Verification items for the finished model (mm, model axes). Face numbers are marked on the shaded views. A direction names the side the tool comes from. Give positions to 0.01 mm unless a question says otherwise; leave off trailing zeros. Order: outer loops, then holes, each group sorted by start corner. A loop starts at its lowest first (then second) coordinate and runs counter-clockwise, first axis right, second up. Notation, with made-up numbers: (-21.5, -20) - (-7.5, -20) arc R27 ccw to (-7.5, 8) - close; hole circle Ø10 at (34, -4.5). An arc over 180 degrees is marked (long way). Answer as a JSON object with one key per item and string values. Group by question number.
(1) Thickness scan on line 1 (Y direction, x = 0, z = 2.4); line 2 (Y direction, x = 0, z = 6); line 3 (Z direction, x = -3.75, y = 1.75). Record the ranges inside material, lowest first.
(2) Section check A-A (x = 0). Record the boundary of the cut face in (y, z), then the cut area to 3 significant figures.
(3) Depth check by flat-ended pin: pin 1 Ø5.5 at (x, y) = (0, 0) entering from +Z; pin 2 Ø2.5 at (x, y) = (-1, 7.5) entering from -Z; pin 3 Ø0.6 at (x, z) = (0.5, 0.5) entering from +Y; pin 4 Ø1 at (x, z) = (0.5, 1) entering from -Y. Enter the tip coordinate at first touch or a pass-through.
(4) Section check C-C (z = 3.75). Record the boundary of the cut face in (x, y).
(5) Section check B-B (z = 1.5). Record the boundary of the cut face in (x, y), then the cut area to 3 significant figures.
(6) Access from +Z, -Z, +X, -X, +Y, -Y to the whole of each face (thin tool, end or side, straight path). Record for the marked faces 1, 2 and 3.
(7) Section check D-D (y = -2.5). Record the boundary of the cut face in (x, z).
(8) Mould release check, pull along Z, two halves, no side actions. Record for the marked faces 4, 5 and 6: +Z half, -Z half, draft (parallel to the pull), parting line (faces both ways), or undercut.
Autodesk Inventor part; units mm, degrees
ref_plane "YZ Plane" through (0, 0, 0) normal (1, 0, 0) x (0, 1, 0)
ref_plane "XZ Plane" through (0, 0, 0) normal (0, 1, 0) x (-1, 0, 0)
ref_plane "XY Plane" through (0, 0, 0) normal (0, 0, 1) x (1, 0, 0)
sketch "Sketch1" plane through (0, 0, 0) normal (0, 0, 1) x (1, 0, 0)
  line L0 (7, 10) -> (-7, 10)
  line L1 (-7, 10) -> (-7, -10)
  line L2 (-7, -10) -> (7, -10)
  line L3 (7, -10) -> (7, 10)
  circle A0 centre (0, 0) radius 3.05
  point P0 (0, -10)
  point P1 (7, 0)
  dimension "d0" = 20
  dimension "d1" = 14
  dimension "d2" = 6.1
extrude "Extrusion1" add sketch "Sketch1" along normal blind 4.4
sketch "Sketch2" plane through (0, 0, 4.4) normal (0, 0, 1) x (1, 0, 0)
  circle A0 centre (0, 0) radius 3 construction
  circle A1 centre (0, 0) radius 7.5 construction
  circle A2 centre (0, 0) radius 3.05 construction
  line L0 (7, 10) -> (-7, 10)
  line L1 (-7, 10) -> (-7, -10)
  line L2 (-7, -10) -> (7, -10)
  line L3 (7, -10) -> (7, 10)
  circle A3 centre (0, 0) radius 7.6
  line L4 (7, -10) -> (7, 10)
  line L5 (7, 2.9597) -> (7, 10)
  line L6 (7, 10) -> (-7, 10)
  line L7 (7, 10) -> (-7, 10)
  line L8 (-7, 10) -> (-7, 2.9597)
  line L9 (-7, 10) -> (-7, -10)
  line L10 (-7, -2.9597) -> (-7, -10)
  line L11 (-7, -10) -> (7, -10)
  line L12 (7, -2.9597) -> (7, -10)
  dimension "d5" = 15.2
extrude "Extrusion2" add sketch "Sketch2" along normal blind 3 contours L3 A3 L1 L0 | L3 L2 L1 A3
sketch "Sketch4" plane through (0, 0, 0) normal (0, 0, -1) x (-1, 0, 0)
  circle A0 centre (0, 7.366) radius 1.15
  circle A1 centre (0, -7.366) radius 1.15
  circle A2 centre (0, 7.366) radius 1.5
  circle A3 centre (0, -7.366) radius 1.5
  point P0 (0, 0)
  dimension "d11" = 3
extrude "Extrusion4" cut sketch "Sketch4" against normal through all contours A0 | A1 | A2 | A3
sketch "Sketch3" plane through (0, 0, 0) normal (0, 0, -1) x (-1, 0, 0)
  circle A0 centre (0, 7.366) radius 1.15 construction
  circle A1 centre (0, -7.366) radius 1.15 construction
  line L0 (2.754, 7.366) -> (1.377, 4.981)
  line L1 (1.377, 4.981) -> (-1.377, 4.981)
  line L2 (-1.377, 4.981) -> (-2.754, 7.366)
  line L3 (-2.754, 7.366) -> (-1.377, 9.751)
  line L4 (-1.377, 9.751) -> (1.377, 9.751)
  line L5 (1.377, 9.751) -> (2.754, 7.366)
  line L6 (1.377, 9.751) -> (1.2332, 10)
  line L7 (-1.377, 9.751) -> (-1.2332, 10)
  line L8 (1.2332, 10) -> (-1.2332, 10)
  line L9 (-7, 10) -> (7, 10)
  point P0 (0, 0)
  dimension "d8" = 4.77
extrude "Extrusion3" cut sketch "Sketch3" against normal blind 2
sketch "Sketch5" plane through (-1.377, 4.981, 0) normal (0, 1, 0) x (1, 0, 0)
  line L0 (-1.377, 0) -> (-1.377, -2) construction
  line L1 (-1.377, 0) -> (-1.377, -1)
  arc A0 (-1.377, -1) -> (-1.377, 0) centre (-1.7436, -0.5) ccw
  point P0 (1.377, 0)
  point P1 (-1.377, -0.5)
  dimension "d15" = 0.62
  dimension "d16" = 0.3666
extrude "Extrusion5" add sketch "Sketch5" along normal blind 3
pattern_circular "Circular Pattern1" count 4 over 180 about axis through (0, 7.366, 0) along (0, 0, 1) of "Extrusion5"
mirror "Mirror1" about plane through (0, 0, 0) normal (0, 1, 0) of "Extrusion3", "Extrusion5", "Circular Pattern1"
chamfer "Chamfer1" distance 2 angle 45 4 edges at (-7, -10, 3.7) (-7, 10, 3.7) (7, 10, 3.7) (7, -10, 3.7)
properties part number "Arm1_BallCasterMount"
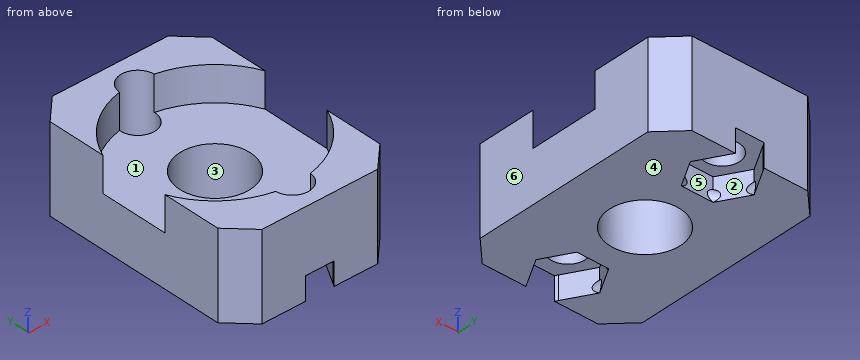
Solutions:
{
 "1": {"line 1": "y = -10 to -8.87, -5.87 to -3.05, 3.05 to 5.87, 8.87 to 10", "line 2": "y = -10 to -8.87, 8.87 to 10", "line 3": "z = 0 to 4.4"},
 "2": {"outline": "(-10, 2) - (-8.87, 2) - (-8.87, 7.4) - (-10, 7.4) - close; (-5.87, 2) - (-4.98, 2) - (-4.98, 0) - (-3.05, 0) - (-3.05, 4.4) - (-5.87, 4.4) - close; (3.05, 0) - (4.98, 0) - (4.98, 2) - (5.87, 2) - (5.87, 4.4) - (3.05, 4.4) - close; (8.87, 2) - (10, 2) - (10, 7.4) - (8.87, 7.4) - close", "area": "33.5 mm2"},
 "3": {"pin 1": "passes through", "pin 2": "stops at z = 2", "pin 3": "stops at y = 4.98", "pin 4": "stops at y = -4.98"},
 "4": {"outline": "(-7, -8) - (-5, -10) - (5, -10) - (7, -8) - (7, 8) - (5, 10) - (-5, 10) - (-7, 8) - close; hole circle Ø6.1 at (0, 0); hole circle Ø3 at (0, -7.37); hole circle Ø3 at (0, 7.37)"},
 "5": {"outline": "(-7, -8) - (-5, -10) - (-1.23, -10) - (-1.38, -9.75) - (-2.75, -7.37) - (-1.38, -4.98) - (1.38, -4.98) - (2.75, -7.37) - (1.38, -9.75) - (1.23, -10) - (5, -10) - (7, -8) - (7, 8) - (5, 10) - (1.23, 10) - (1.38, 9.75) - (2.75, 7.37) - (1.38, 4.98) - (-1.38, 4.98) - (-2.75, 7.37) - (-1.38, 9.75) - (-1.23, 10) - (-5, 10) - (-7, 8) - close; hole circle Ø6.1 at (0, 0)", "area": "202 mm2"},
 "6": {"face 1": "+Z", "face 2": "none", "face 3": "+Z, -Z"},
 "7": {"outline": "(-7, 0) - (-1.75, 0) - (-1.75, 4.4) - (-7, 4.4) - close; (1.75, 0) - (7, 0) - (7, 4.4) - (1.75, 4.4) - close"},
 "8": {"face 4": "-Z half", "face 5": "undercut", "face 6": "draft"}
}
